The figure shows three views and two pictorial views of one solid part (mm, origin at its lowest corner). Answer the questions. A direction names the side the tool comes from. Round coordinates to 2 decimals unless told otherwise and drop trailing zeros. Loops run counter-clockwise (first coordinate to the right, second up) from the corner with the lowest first, then second, coordinate; pieces in that order, holes last. Notation, with made-up numbers: (76, 86.5) -> (127, 86.5) arc R19 cw to (127, 122.5) -> close; hole circle Ø8 at (45.5, -3.75). An arc over 180 degrees is marked (long way). Put each result on its own line as item: value.
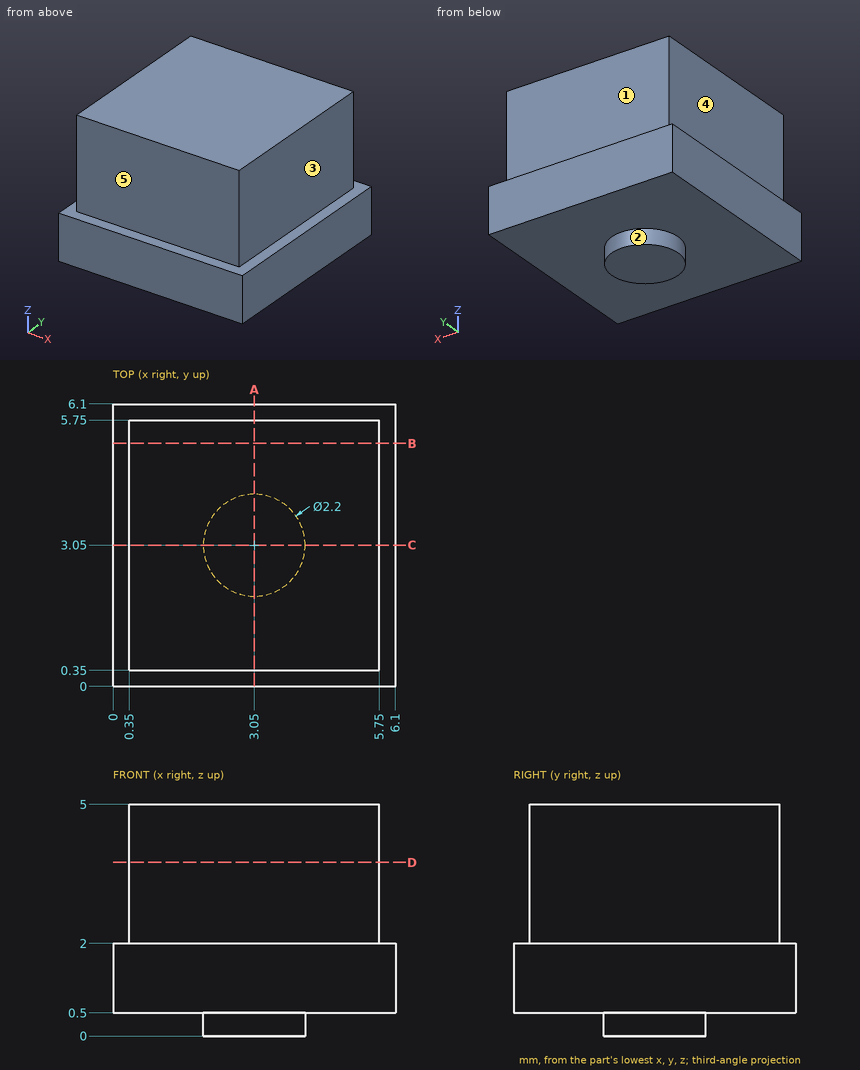
Item 1: Find the intervals of material crossed by line 1 along Z through (x, y) = (4.75, 4.5); line 2 along Y through (x, z) = (0.75, 3.35), in increasing order.
Derived:
line 1: z = 0.5 to 5
line 2: y = 0.35 to 5.75
Item 2: The part is cut by section A-A (x = 3.05). Determine the outline of the cut face in (y, z), then the cut area to 4 significant figures.
Derived:
outline: (0, 0.5) -> (1.95, 0.5) -> (1.95, 0) -> (4.15, 0) -> (4.15, 0.5) -> (6.1, 0.5) -> (6.1, 2) -> (5.75, 2) -> (5.75, 5) -> (0.35, 5) -> (0.35, 2) -> (0, 2) -> close
area: 26.45 mm^2
Item 3: The part is cut by section D-D (z = 3.75). Determine the outline of the cut face in (x, y).
Derived:
outline: (0.35, 0.35) -> (5.75, 0.35) -> (5.75, 5.75) -> (0.35, 5.75) -> close
Item 4: Flat-ended cylindrical pins translate along their axes: pin 1 Ø1 at (y, z) = (4, 3.5) entering from +X; pin 2 Ø0.9 at (y, z) = (3, 4) entering from -X; pin 3 Ø1.5 at (x, z) = (4, 3.5) entering from +Y. Find the tip coordinate at first contact, or state that the pin passes through.
Derived:
pin 1: stops at x = 5.75
pin 2: stops at x = 0.35
pin 3: stops at y = 5.75
Item 5: Which of the six approach directions +Z, -Z, +X, -X, +Y, -Y give full straight-line access (tool end or side, diameter ignored) to the marked faces 1, 2, 3, 4 and 5?
Derived:
face 1: +Z, +X, -X, +Y
face 2: -Z
face 3: +Z, +X, +Y, -Y
face 4: +Z, -X, +Y, -Y
face 5: +Z, +X, -X, -Y
Item 6: The part is cut by section B-B (y = 5.25). Determine the outline of the cut face in (x, z), then the cut area to 4 significant figures.
Derived:
outline: (0, 0.5) -> (6.1, 0.5) -> (6.1, 2) -> (5.75, 2) -> (5.75, 5) -> (0.35, 5) -> (0.35, 2) -> (0, 2) -> close
area: 25.35 mm^2
